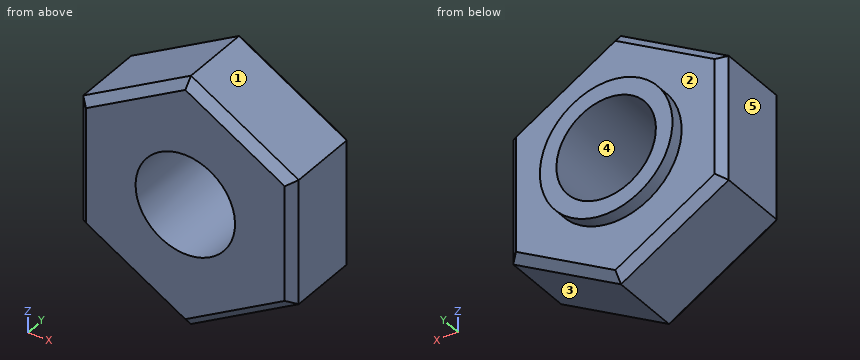
```python
from build123d import *

# Parameters (mm, degrees)
SKETCH1_R           = 3
BOSS_EXTRUDE1_DEPTH = 6
SKETCH3_R           = 4
CUT_EXTRUDE1_DEPTH  = 0.8
CHAMFER1_SIZE       = 0.5


with BuildPart() as part:
    # Sketch1 → Boss-Extrude1 (new body)
    with BuildSketch(Plane(origin=(0, 0, 0), x_dir=(1, 0, 0), z_dir=(0, 1, 0))):
        Polygon((0, -7.505553499), (6.5, -3.75277675), (6.5, 3.75277675), (0, 7.505553499), (-6.5, 3.75277675), (-6.5, -3.75277675), align=None)
        with Locations(Location((0, 0, 0), (0, 0, 270))):
            Circle(SKETCH1_R, mode=Mode.SUBTRACT)
    extrude(amount=BOSS_EXTRUDE1_DEPTH)

    # Sketch3 → Cut-Extrude1 (cut)
    with BuildSketch(Plane(origin=(0, 6, 0), x_dir=(1, 0, 0), z_dir=(0, 1, 0))):
        Polygon((-6.5, -3.75277675), (0, -7.505553499), (6.5, -3.75277675), (6.5, 3.75277675), (0, 7.505553499), (-6.5, 3.75277675), align=None)
        with Locations(Location((0, 0, 0), (0, 0, 270))):
            Circle(SKETCH3_R, mode=Mode.SUBTRACT)
    extrude(amount=-CUT_EXTRUDE1_DEPTH, mode=Mode.SUBTRACT)

    # Chamfer1
    chamfer1_edges = [part.edges().sort_by_distance(p)[0] for p in [
        (-6.5, 5.2, 0),
        (-3.25, 5.2, -5.629165125),
        (3.25, 5.2, -5.629165125),
        (6.5, 5.2, 0),
        (3.25, 5.2, 5.629165125),
        (-3.25, 5.2, 5.629165125),
        (-6.5, 0, 0),
        (-3.25, 0, -5.629165125),
        (3.25, 0, -5.629165125),
        (6.5, 0, 0),
        (3.25, 0, 5.629165125),
        (-3.25, 0, 5.629165125),
    ]]
    chamfer(chamfer1_edges, length=CHAMFER1_SIZE)


solid = part.part
```
Verification items for the finished model (mm, model axes). Face numbers are marked on the shaded views. A direction names the side the tool comes from. Round coordinates to 2 decimals unless told otherwise and drop trailing zeros. Order: outer loops, then holes, each group sorted by start corner. A loop starts at its lowest first (then second) coordinate and runs counter-clockwise, first axis right, second up.
1) Cross-section at D-D, the plane z = -5.25. Record the cut outline in (x, y).
Geometry says:
outline: (-3.91, 0.5) - (-2.91, 0) - (2.91, 0) - (3.91, 0.5) - (3.91, 4.7) - (2.91, 5.2) - (-2.91, 5.2) - (-3.91, 4.7) - close
2) Draft check along Z on the marked faces 3, 4 and 5. Enter one of: +Z half, -Z half, draft (parallel to the pull), parting line (faces both ways), or undercut.
Geometry says:
face 3: -Z half
face 4: undercut
face 5: draft
3) Cross-section at A-A, the plane y = 4. Record the cut outline in (x, z).
Geometry says:
outline: (-6.5, -3.75) - (0, -7.51) - (6.5, -3.75) - (6.5, 3.75) - (0, 7.51) - (-6.5, 3.75) - close; hole circle Ø6 at (0, 0)
4) Material ranges on line 1 (X direction, y = 3, z = 0); line 2 (Z direction, x = 0.5, y = 5); line 3 (Z direction, x = -1, y = 5.5), recorded low to high.
Geometry says:
line 1: x = -6.5 to -3, 3 to 6.5
line 2: z = -6.87 to -2.96, 2.96 to 6.87
line 3: z = -3.87 to -2.83, 2.83 to 3.87
5) Depth check by flat-ended pin: pin 1 (3 mm diameter, centred on x = -5, y = 5.5, fed in from +Z); pin 2 (5 mm diameter, centred on x = 3.5, z = 3, fed in from +Y); pin 3 (3.5 mm diameter, centred on x = 0, z = 0, fed in from +Y) (3 decimals); pin 4 (3 mm diameter, centred on x = -2.5, z = 5, fed in from +Y). Enter the tip coordinate at first touch or a pass-through.
Geometry says:
pin 1: stops at z = 5.35
pin 2: stops at y = 6
pin 3: passes through
pin 4: stops at y = 5.2
6) Cross-section at B-B, the plane z = 0. Record the cut outline in (x, y).
Geometry says:
outline: (-6.5, 0.5) - (-6, 0) - (-3, 0) - (-3, 6) - (-4, 6) - (-4, 5.2) - (-6, 5.2) - (-6.5, 4.7) - close; (3, 0) - (6, 0) - (6.5, 0.5) - (6.5, 4.7) - (6, 5.2) - (4, 5.2) - (4, 6) - (3, 6) - close
7) Cross-section at C-C, the plane x = 2. Record the cut outline in (y, z), plus the area to 3 significant figures.
Geometry says:
outline: (0, -5.77) - (0.5, -6.35) - (4.7, -6.35) - (5.2, -5.77) - (5.2, -3.46) - (6, -3.46) - (6, -2.24) - (0, -2.24) - close; (0, 2.24) - (6, 2.24) - (6, 3.46) - (5.2, 3.46) - (5.2, 5.77) - (4.7, 6.35) - (0.5, 6.35) - (0, 5.77) - close
area: 44.2 mm2
8) Tool access check on the marked faces 1 and 2. Record the directions out of +Z, -Z, +X, -X, +Y, -Y that give a thin tool (end or side, any length) a straight path to the whole face; none if there is none.
Geometry says:
face 1: +Z, +X, +Y, -Y
face 2: +Y
